Design review of the part built by this model. Coordinates are the model's own, in mm. A direction names the side the tool comes from. Coordinates: 2 decimals unless noted, no trailing zeros. Write each loop counter-clockwise with the first axis right and the second up, starting at its lowest first coordinate (ties: lowest second). Pieces come first, ordered by that corner, then holes. Notation, with made-up numbers: M -11.5,87.25 L 13.5,87.25 A8 cw 13.5,94.25 Z; hole C -6,-10.5 d6. An arc over 180 degrees is marked long. Write item = value, one per line.
Autodesk Inventor part; units mm, degrees
ref_plane "YZ Plane" through (0, 0, 0) normal (1, 0, 0) x (0, 1, 0)
ref_plane "XZ Plane" through (0, 0, 0) normal (0, 1, 0) x (-1, 0, 0)
ref_plane "XY Plane" through (0, 0, 0) normal (0, 0, 1) x (1, 0, 0)
sketch "Sketch1" plane through (0, 0, 0) normal (0, 0, 1) x (1, 0, 0)
  line L0 (0, 0) -> (20, 0)
  line L1 (20, 0) -> (20, 120)
  line L2 (0, 0) -> (0, 120)
  line L3 (0, 0) -> (120, 0) construction
  line L4 (20, 120) -> (22.1131, 124.5315)
  line L5 (20, 120) -> (25, 120) construction
  line L6 (0, 120) -> (-2.1131, 124.5315)
  line L7 (-2.1131, 124.5315) -> (-2.1131, 149.5315)
  line L8 (-2.1131, 149.5315) -> (22.1131, 149.5315)
  line L9 (22.1131, 149.5315) -> (22.1131, 124.5315)
  dimension "d0" = 20
  dimension "d1" = 120
  dimension "d2" = 90
  dimension "d3" = 120
  dimension "d4" = 90
  dimension "d5" = 5
  dimension "d6" = 65
  dimension "d7" = 5
  dimension "d8" = 25
extrude "Extrusion1" add sketch "Sketch1" along normal blind 5
sketch "Sketch2" plane through (0, 0, 5) normal (0, 0, 1) x (1, 0, 0)
  point P0 (0, 0)
  point P1 (10, 10)
hole "Hole1" at (10, 10, 5) direction (0, 0, -1) diameter 3 end through all
sketch "Sketch3" plane through (0, 0, 5) normal (0, 0, 1) x (1, 0, 0)
  point P0 (0, 0)
sketch "Sketch4" plane through (0, 0, 5) normal (0, 0, 1) x (1, 0, 0)
  point P0 (0, 0)
  point P1 (10, 75)
hole "Hole2" at (10, 75, 5) direction (0, 0, -1) diameter 3 end through all
sketch "Sketch5" plane through (0, 0, 5) normal (0, 0, 1) x (1, 0, 0)
  circle A0 centre (10, 10) radius 1.5
  line L0 (11.4716, 74.9905) -> (8.5, 74.9905)
  line L1 (8.5, 74.9905) -> (8.5, 10)
  line L2 (8.5, 10) -> (11.4716, 10)
  line L3 (11.4716, 10) -> (11.4716, 74.9905)
  point P0 (0, 0)
extrude "Extrusion2" cut sketch "Sketch5" against normal blind 10 contours L1 L0 L3 A0 | A0 L3 L2 picked at (9.5055, 10.1215)
sketch "Sketch6" plane through (0, 0, 5) normal (0, 0, 1) x (1, 0, 0)
  point P0 (0, 0)
  point P1 (10, 85)
hole "Hole3" at (10, 85, 5) direction (0, 0, -1) diameter 3 end through all
sketch "Sketch8" plane through (0, 0, 0) normal (0, 0, -1) x (-1, 0, 0)
  point P0 (0, 0)
  point P1 (-10, -8)
hole "Hole4" at (10, -8, 0) direction (0, 0, 1) diameter 3 end through all
sketch "Sketch10" plane through (0, 0, 5) normal (0, 0, 1) x (1, 0, 0)
  line L0 (22.1131, 124.5315) -> (22.1131, 149.5315)
  line L1 (-2.1131, 149.5315) -> (-2.1131, 124.5315)
  point P0 (0, 0)
  dimension "d45" = 24.2262
sketch "Sketch11" plane through (0, 0, 5) normal (0, 0, 1) x (1, 0, 0)
  point P0 (0, 0)
sketch "Sketch12" plane through (0, 0, 5) normal (0, 0, 1) x (1, 0, 0)
  point P0 (0, 0)
sketch "Sketch13" plane through (0, 0, 5) normal (0, 0, 1) x (1, 0, 0)
  point P0 (0, 0)
properties material "Steel, Cast"
Q1. Consider section D-D, the plane y = 69.5. State the section outline as (x, z) points.
Check result:
outline = M 0,0 L 8.5,0 L 8.5,5 L 0,5 Z; M 11.47,0 L 20,0 L 20,5 L 11.47,5 Z
Q2. Wall thickness on line 1 (Y direction, x = 10, z = 2.45); line 2 (X direction, y = 10, z = 2.1); line 3 (Y direction, x = 9.25, z = 4): over which ranges is each line inside the solid? List them lowest first.
Check result:
line_1 = 0 to 8.5, 76.5 to 83.5, 86.5 to 149.53
line_2 = 0 to 8.5, 11.5 to 20
line_3 = 0 to 8.7, 76.3 to 83.7, 86.3 to 149.53
Q3. Consider section C-C, the plane z = 3.1. State how many separate pieces and enclosed holes the cut face has, and give its area (3 significant figures).
Check result:
separate_pieces = 1
enclosed_holes = 2
area = 2,900 mm²
Q4. For P1, Ø2.5, axis at x = 10, y = 85, coming from the -Z side; P2, Ø3, axis at x = 3.5, y = 73, coming from the -Z side; P3, Ø3, axis at y = 76, z = 3, coming from the +X side; P4, Ø1.5, axis at y = 55, z = 3.5, coming from the -X side, all flat-tipped, find the tip position at first contact; note any pin that passes through.
Check result:
P1 = through
P2 = 0
P3 = 20
P4 = 0
Q5. Consider section A-A, the plane y = 85. State the section outline as (x, z) points.
Check result:
outline = M 0,0 L 8.5,0 L 8.5,5 L 0,5 Z; M 11.5,0 L 20,0 L 20,5 L 11.5,5 Z
Q6. Machinability: for faces 1 (the flat face through (11.472, 42, 3)), 2 (the flat face through (20, 59, 2)), 3 (the flat face through (0, 59, 2)), 4 (the flat face through (7, 76, 5)), which of the approach directions +Z, -Z, +X, -X, +Y, -Y give a long, thin tool a straight path to every point of the face, cutting with its end or side? Answer none if there is none.
Check result:
face_1 = +Z, -Z
face_2 = +Z, -Z, +X, -Y
face_3 = +Z, -Z, -X, -Y
face_4 = +Z, +X, -X, +Y, -Y
Q7. Consider section B-B, the plane x = 10. State the section outline as (y, z) points, and give its area (3 significant figures).
Check result:
outline = M 0,0 L 8.5,0 L 8.5,5 L 0,5 Z; M 76.5,0 L 83.5,0 L 83.5,5 L 76.5,5 Z; M 86.5,0 L 149.53,0 L 149.53,5 L 86.5,5 Z
area = 393 mm²
Q8. The part is to be moulded in two halves that separate along X. For faces 5 (the cylindrical face through (10.575, 83.614, 2.465)), 6 (the flat face through (10, 0, 2)), 7 (the flat face through (-1.04, 122.23, 2.46)), say which applies: +X half, -X half, draft (parallel to the pull), parting line (faces both ways), or undercut.
Check result:
face_5 = undercut
face_6 = draft
face_7 = -X half
